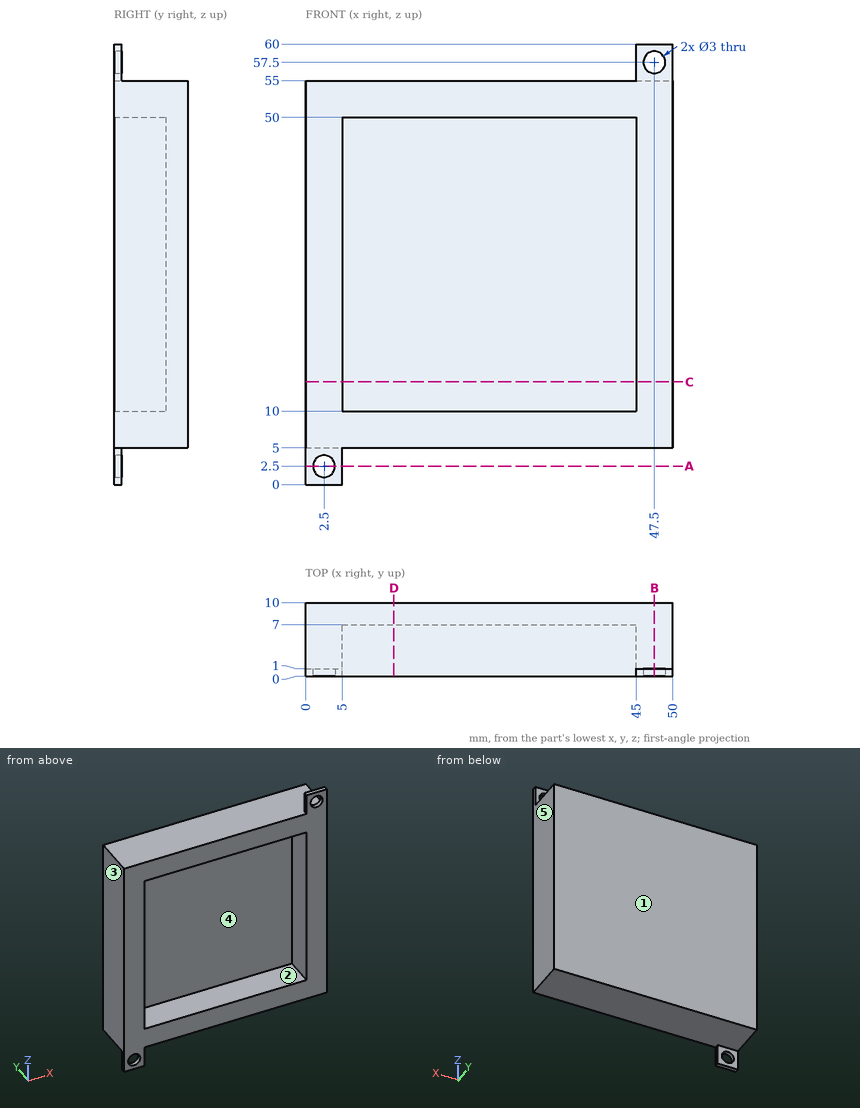
For this review, use the dimensioned drawing (mm, ordinates from the lowest corner) and the shaded views. A direction names the side the tool comes from. Round coordinates to 2 decimals unless told otherwise and drop trailing zeros. Order: outer loops, then holes, each group sorted by start corner. A loop starts at its lowest first (then second) coordinate and runs counter-clockwise, first axis right, second up. Notation, with made-up numbers: (65.25, 45) -> (73.25, 45) arc R35 cw to (73.25, 77) -> close; hole circle Ø10 at (85, -5). An arc over 180 degrees is marked (long way). Write item = value, one per line. Start each with the question number.
Item 1: Clearance check with flat-ended pins moving along their axes: pin 1 Ø3.5 at (x, y) = (29, 2) entering from +Z; pin 2 Ø2.5 at (x, z) = (1.5, 3) entering from +Y; pin 3 Ø1.5 at (x, z) = (47.5, 58) entering from +Y; pin 4 Ø1 at (x, y) = (44, 6.5) entering from -Z. State where each tip first meets the part, or that it passes through.
Item 2: Mouldability with a two-part tool opening along X and no side actions: class the marked faces 1, 2 and 3 as released by +X, released by -X, zero draft, split by the parting line, or undercut.
Item 3: Consider section D-D on x = 12. Write out the cut boundary in (y, z).
Item 4: Consider section B-B on x = 47.5. Write out the cut boundary in (y, z), plus the area to 3 significant figures.
Item 5: For line 1 along X through (y, z) = (3.75, 27); line 2 along X through (y, z) = (0.85, 57.5); line 3 along Z through (x, y) = (20, 1.5), list the stretches that pass through material, from the lowest coordinate up.
Item 6: Consider section C-C on z = 14. Write out the cut boundary in (x, y).
Item 7: Consider section A-A on z = 2.5. Write out the cut boundary in (x, y), plus the area to 3 significant figures.
Item 8: For the marked faces 4 and 5, list the 3-axis set-ups (+Z, -Z, +X, -X, +Y, -Y) from which the entire face can be reached by the end or side of a thin tool; tool diameter is ignored.
Conclusion:
q1.pin_1 = 55
q1.pin_2 = 1
q1.pin_3 = through
q1.pin_4 = 5
q2.face_1 = zero draft
q2.face_2 = undercut
q2.face_3 = released by -X
q3.outline = (0, 5) -> (10, 5) -> (10, 55) -> (0, 55) -> (0, 50) -> (7, 50) -> (7, 10) -> (0, 10) -> close
q4.outline = (0, 5) -> (10, 5) -> (10, 55) -> (1, 55) -> (1, 56) -> (0, 56) -> close; (0, 59) -> (1, 59) -> (1, 60) -> (0, 60) -> close
q4.area = 502 mm2
q5.line_1 = 0 to 5, 45 to 50
q5.line_2 = 45 to 46, 49 to 50
q5.line_3 = 5 to 10, 50 to 55
q6.outline = (0, 0) -> (5, 0) -> (5, 7) -> (45, 7) -> (45, 0) -> (50, 0) -> (50, 10) -> (0, 10) -> close
q7.outline = (0, 0) -> (1, 0) -> (1, 1) -> (0, 1) -> close; (4, 0) -> (5, 0) -> (5, 1) -> (4, 1) -> close
q7.area = 2.00 mm2
q8.face_4 = -Y
q8.face_5 = +Z, -Z, +X, +Y, -Y
